The drawing under review shows one solid part. Ordinate dimensions are in mm from its lowest x, y, z. Coordinates: 2 decimals unless noted, no trailing zeros. Order: outer loops, then holes, each group sorted by start corner. A loop starts at its lowest first (then second) coordinate and runs counter-clockwise, first axis right, second up. Notation, with made-up numbers: (41, 62) - (95, 62) arc R21 ccw to (95, 95) - close; hole circle Ø10 at (31, -24.5). An arc over 180 degrees is marked (long way). Write each question's results on one line, items separated by ' | '. Start each with the question number.
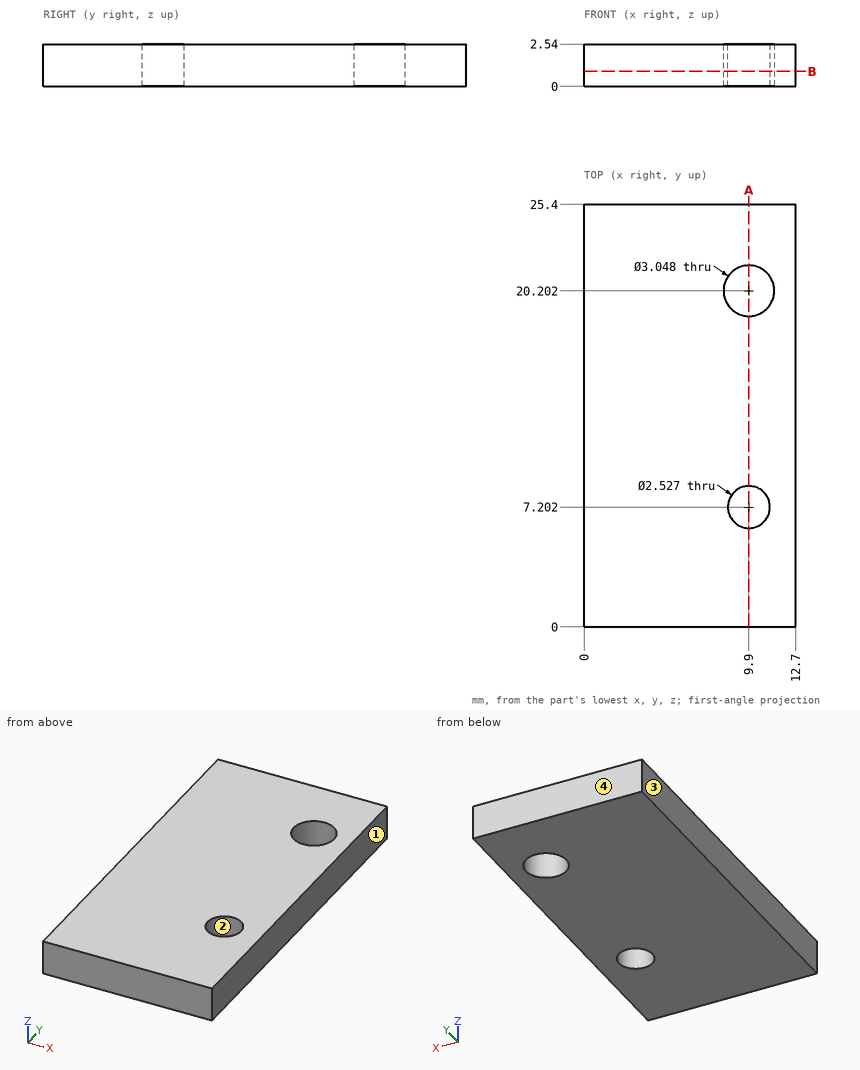
(1) Take a section at A-A (x = 9.9). State the section outline as (y, z) points (1 decimal).
(2) Take a section at B-B (z = 0.9). State the section outline as (x, y) points, plus the area to 3 significant figures.
(3) To check wall thickness, follow line 1 along Y through (x, z) = (9.9, 0.7) (1 decimal); line 2 along Y through (x, z) = (8.75, 0.15) (1 decimal); line 3 along X through (y, z) = (6.5, 0.8). State the ranges of each line that lie inside material, in increasing order. Write a range as [from, to].
(4) Mouldability with a two-part tool opening along X and no side actions: class the marked faces 1, 2, 3 and 4 as +X half, -X half, draft (parallel to the pull), parting line (faces both ways), or undercut.
Worked out:
1) outline: (0, 0) - (5.9, 0) - (5.9, 2.5) - (0, 2.5) - close; (8.5, 0) - (18.7, 0) - (18.7, 2.5) - (8.5, 2.5) - close; (21.7, 0) - (25.4, 0) - (25.4, 2.5) - (21.7, 2.5) - close
2) outline: (0, 0) - (12.7, 0) - (12.7, 25.4) - (0, 25.4) - close; hole circle Ø3.05 at (9.9, 20.2); hole circle Ø2.53 at (9.9, 7.2) | area: 310 mm^2
3) line 1: [0, 5.9], [8.5, 18.7], [21.7, 25.4] | line 2: [0, 6.7], [7.7, 19.2], [21.2, 25.4] | line 3: [0, 8.85], [10.95, 12.7]
4) face 1: +X half | face 2: undercut | face 3: -X half | face 4: draft
